```python
from build123d import *

# Parameters (mm, degrees)
SKETCH1_W           = 61
SKETCH1_H           = 100
BOSS_EXTRUDE1_DEPTH = 3
SKETCH3_R           = 1.5
BOSS_EXTRUDE7_DEPTH = 3
LPATTERN1_COUNT     = 2
LPATTERN1_PITCH     = 15
SKETCH6_W           = 5
SKETCH6_H           = 8
CUT_EXTRUDE1_DEPTH  = 5
SKETCH4_W           = 61
SKETCH4_H           = 3
BOSS_EXTRUDE3_DEPTH = 10
SKETCH8_R           = 0.5
BOSS_EXTRUDE6_DEPTH = 3
SKETCH9_W           = 3
SKETCH9_H           = 3
CUT_EXTRUDE3_DEPTH  = 3


with BuildPart() as part:
    # Sketch1 → Boss-Extrude1 (new body)
    with BuildSketch(Plane(origin=(0, 0, 0), x_dir=(1, 0, 0), z_dir=(0, 1, 0))):
        with Locations((30.5, 50)):
            Rectangle(SKETCH1_W, SKETCH1_H)
    extrude(amount=BOSS_EXTRUDE1_DEPTH)

    # Sketch3 → Boss-Extrude7 (add)
    with BuildSketch(Plane(origin=(24.5, 0, 0), x_dir=(0, 0, -1), z_dir=(1, 0, 0))):
        Circle(SKETCH3_R)
    boss_extrude7 = extrude(amount=-BOSS_EXTRUDE7_DEPTH)

    # LPattern1: Boss-Extrude7 ×2
    with Locations(*[(i * LPATTERN1_PITCH, 0, 0) for i in range(1, LPATTERN1_COUNT)]):
        add(boss_extrude7)

    # Sketch6 → Cut-Extrude1 (cut)
    with BuildSketch(Plane(origin=(0, 3, 0), x_dir=(1, 0, 0), z_dir=(0, 1, 0))):
        with Locations((55.5, 7)):
            Rectangle(SKETCH6_W, SKETCH6_H)
    extrude(amount=-CUT_EXTRUDE1_DEPTH, mode=Mode.SUBTRACT)

    # Sketch4 → Boss-Extrude3 (add)
    with BuildSketch(Plane.XY):
        with Locations((30.5, 1.5)):
            Rectangle(SKETCH4_W, SKETCH4_H)
    extrude(amount=BOSS_EXTRUDE3_DEPTH)

    # Sketch8 → Boss-Extrude6 (add)
    with BuildSketch(Plane(origin=(61, 0, 0), x_dir=(0, 0, -1), z_dir=(1, 0, 0))):
        with BuildLine():
            Line((13.5, 3), (16.5, 3))
            Line((16.5, 3), (16.5, 5))
            ThreePointArc((16.5, 5), (15, 6.5), (13.5, 5))
            Line((13.5, 5), (13.5, 3))
        make_face()
        with Locations(Location((15, 5, 0), (0, 0, 180))):
            Circle(SKETCH8_R, mode=Mode.SUBTRACT)
    extrude(amount=-BOSS_EXTRUDE6_DEPTH)

    # Sketch9 → Cut-Extrude3 (cut)
    with BuildSketch(Plane.XZ):
        with Locations((35, 0)):
            Rectangle(SKETCH9_W, SKETCH9_H)
        with Locations((26, 0)):
            Rectangle(SKETCH9_W, SKETCH9_H)
    extrude(amount=-CUT_EXTRUDE3_DEPTH, mode=Mode.SUBTRACT)


solid = part.part
```
Verification items for the finished model (mm, model axes). A direction names the side the tool comes from. Coordinates: 2 decimals unless noted, no trailing zeros. Loops run counter-clockwise (first coordinate to the right, second up) from the corner with the lowest first, then second, coordinate; pieces in that order, holes last. Notation, with made-up numbers: (40.25, 52) - (88.25, 52) arc R20 ccw to (88.25, 83) - close; hole circle Ø7 at (0, -14.75). An arc over 180 degrees is marked (long way). Answer as a JSON object with one key per item and string values.
(1) Mould release check, pull along X, two halves, no side actions. Record for faces 1 (the flat face through (58, 4, -15)), 2 (the flat face through (53, 2, -7)), 3 (the cylindrical face through (38, -1.5, 0)): pulls with the +X half, pulls with the -X half, needs draft (parallel to the pull), parting line crosses it, or undercut.
Response:
{"face 1": "pulls with the -X half", "face 2": "undercut", "face 3": "needs draft"}
(2) Access from +Z, -Z, +X, -X, +Y, -Y to the whole of each face (thin tool, end or side, straight path). Record for faces 4 (the flat face through (30, 2, 10)), 5 (the flat face through (60, 4, -13.5)), 6 (the flat face through (60, 4, -16.5)), 7 (the flat face through (26, 1, 1.5)).
Response:
{"face 4": "+Z, +X, -X, +Y, -Y", "face 5": "+Z, +X, -X, +Y", "face 6": "-Z, +X, -X, +Y", "face 7": "+Y, -Y"}
(3) Cross-section at A-A, the plane z = -6. Record the boundary of the cut face in (x, y).
Response:
{"outline": "(0, 0) - (53, 0) - (53, 3) - (0, 3) - close; (58, 0) - (61, 0) - (61, 3) - (58, 3) - close"}
(4) Scan lines: line 1 along Y through (x, z) = (59, -15); line 2 along X through (y, z) = (1, -8); line 3 along Z through (x, y) = (59.3, 5). Record each from-to range of solid material in increasing order.
Response:
{"line 1": "y = 0 to 4.5, 5.5 to 6.5", "line 2": "x = 0 to 53, 58 to 61", "line 3": "z = -16.5 to -15.5, -14.5 to -13.5"}
(5) Cross-section at B-B, the plane x = 11. Record the boundary of the cut face in (y, z), then the cut area to 3 significant figures.
Response:
{"outline": "(0, -100) - (3, -100) - (3, 10) - (0, 10) - close", "area": "330 mm²"}
(6) Cross-section at C-C, the plane z = -86. Record the boundary of the cut face in (x, y), then the cut area to 3 significant figures.
Response:
{"outline": "(0, 0) - (61, 0) - (61, 3) - (0, 3) - close", "area": "183 mm²"}
(7) Go/stop test with flat-tipped pins: pin 1 Ø0.5 at (y, z) = (-1, 0) entering from -X; pin 2 Ø8 at (x, z) = (27.5, -65) entering from -Y; pin 3 Ø1.7 at (y, z) = (-1, 0.5) entering from +X. Record where each tip stops, or that it passes through.
Response:
{"pin 1": "stops at x = 21.5", "pin 2": "stops at y = 0", "pin 3": "stops at x = 39.5"}
